from build123d import *

# Parameters (mm, degrees)
SKETCH1_W           = 127
SKETCH1_H           = 127
BOSS_EXTRUDE1_DEPTH = 127
SKETCH13_W          = 43.18
SKETCH13_H          = 43.18
SKETCH13_W_2        = 29.718
SKETCH13_H_2        = 29.718
BOSS_EXTRUDE7_DEPTH = 6.35
SKETCH29_R          = 40.64
CUT_EXTRUDE10_DEPTH = 6.35
SKETCH27_W          = 43.18
SKETCH27_H          = 43.18
SKETCH27_W_2        = 29.718
SKETCH27_H_2        = 29.718
BOSS_EXTRUDE8_DEPTH = 6.35
SKETCH28_R          = 40.64
CUT_EXTRUDE11_DEPTH = 6.35


with BuildPart() as part:
    # Sketch1 → Boss-Extrude1 (new body)
    with BuildSketch(Plane.XY):
        Rectangle(SKETCH1_W, SKETCH1_H)
    extrude(amount=BOSS_EXTRUDE1_DEPTH)

    # Sketch13 → Boss-Extrude7 (add)
    with BuildSketch(Plane(origin=(0, 0, 0), x_dir=(-1, 0, 0), z_dir=(0, 0, -1))):
        with Locations((-41.91, 41.91)):
            Rectangle(SKETCH13_W, SKETCH13_H)
        with Locations((-41.91, -41.91)):
            Rectangle(SKETCH13_W, SKETCH13_H)
        with Locations((41.91, 41.91)):
            Rectangle(SKETCH13_W, SKETCH13_H)
        with Locations((41.91, -41.91)):
            Rectangle(SKETCH13_W, SKETCH13_H)
        with Locations((-48.641, 0)):
            Rectangle(SKETCH13_W_2, SKETCH13_H_2)
        with Locations((0, -48.641)):
            Rectangle(SKETCH13_W_2, SKETCH13_H_2)
        with Locations((48.641, 0)):
            Rectangle(SKETCH13_W_2, SKETCH13_H_2)
        with Locations((0, 48.641)):
            Rectangle(SKETCH13_W_2, SKETCH13_H_2)
    extrude(amount=BOSS_EXTRUDE7_DEPTH)

    # Sketch29 → Cut-Extrude10 (cut)
    with BuildSketch(Plane(origin=(0, 0, 0), x_dir=(-1, 0, 0), z_dir=(0, 0, -1))):
        Circle(SKETCH29_R)
    extrude(amount=CUT_EXTRUDE10_DEPTH, mode=Mode.SUBTRACT)

    # Sketch27 → Boss-Extrude8 (add)
    with BuildSketch(Plane(origin=(63.5, 0, 0), x_dir=(0, 0, -1), z_dir=(1, 0, 0))):
        with Locations((-105.41, 41.91)):
            Rectangle(SKETCH27_W, SKETCH27_H)
        with Locations((-105.41, -41.91)):
            Rectangle(SKETCH27_W, SKETCH27_H)
        with Locations((-21.59, 41.91)):
            Rectangle(SKETCH27_W, SKETCH27_H)
        with Locations((-21.59, -41.91)):
            Rectangle(SKETCH27_W, SKETCH27_H)
        with Locations((-112.141, -0.254760407)):
            Rectangle(SKETCH27_W_2, SKETCH27_H_2)
        with Locations((-63.013602448, -48.641)):
            Rectangle(SKETCH27_W_2, SKETCH27_H_2)
        with Locations((-14.859, -0.254760407)):
            Rectangle(SKETCH27_W_2, SKETCH27_H_2)
        with Locations((-63.013602448, 48.641)):
            Rectangle(SKETCH27_W_2, SKETCH27_H_2)
    extrude(amount=BOSS_EXTRUDE8_DEPTH)

    # Sketch28 → Cut-Extrude11 (cut)
    with BuildSketch(Plane(origin=(63.5, 0, 0), x_dir=(0, 0, -1), z_dir=(1, 0, 0))):
        with Locations((-63.5, 0)):
            Circle(SKETCH28_R)
    extrude(amount=CUT_EXTRUDE11_DEPTH, mode=Mode.SUBTRACT)


solid = part.part
Can you work these out from the model? Positions are in its coordinate system, mm. A direction names the side the tool comes from. Give positions to 0.01 mm unless a question says otherwise; leave off trailing zeros. Order: outer loops, then holes, each group sorted by start corner. A loop starts at its lowest first (then second) coordinate and runs counter-clockwise, first axis right, second up. Notation, with made-up numbers: M -3,86 L 48,86 A21 cw 48,107 Z; hole C 36,22 d3. An arc over 180 degrees is marked long. One line per item, written item: value.
Item 1: If we section it at C-C on z = 54: Write out the boundary of the cut face in (x, y).
Verdict:
outline: M -63.5,-63.5 L 69.85,-63.5 L 69.85,-39.51 L 63.5,-39.51 L 63.5,39.51 L 69.85,39.51 L 69.85,63.5 L -63.5,63.5 Z
Item 2: For pin 1 (3 mm diameter, centred on y = -38, z = -4, fed in from +X); pin 2 (12 mm diameter, centred on x = 15.5, y = 22.5, fed in from -Z), each with a flat end and sliding along its axis, tell me the tip position at first contact or that it passes through.
Verdict:
pin 1: x = 63.5
pin 2: z = 0
Item 3: If we mould it in two halves opening along Y, with no side actions, what happens to faces 5 (the face through (-49, 20.32, -3)), 6 (the face through (69.85, -50, 63))? For each: pulls with the +Y half, pulls with the -Y half, needs draft (parallel to the pull), parting line crosses it, or undercut.
Verdict:
face 5: undercut
face 6: needs draft
Item 4: If we section it at A-A on y = -9.5: Write out the boundary of the cut face in (x, z).
Verdict:
outline: M -63.5,-6.35 L -39.51,-6.35 L -39.51,0 L 39.51,0 L 39.51,-6.35 L 63.5,-6.35 L 63.5,0 L 69.85,0 L 69.85,23.99 L 63.5,23.99 L 63.5,103.01 L 69.85,103.01 L 69.85,127 L -63.5,127 Z
Item 5: If we section it at D-D on y = 26: Write out the boundary of the cut face in (x, z).
Verdict:
outline: M -63.5,-6.35 L -31.23,-6.35 L -31.23,0 L 31.23,0 L 31.23,-6.35 L 63.5,-6.35 L 63.5,0 L 69.85,0 L 69.85,32.27 L 63.5,32.27 L 63.5,94.73 L 69.85,94.73 L 69.85,127 L -63.5,127 Z
Item 6: Please list where these lines run through material, in increasing order: line 1 (Z direction, x = 4, y = 24); line 2 (X direction, y = 3.5, z = 59).
Verdict:
line 1: 0 to 127
line 2: -63.5 to 63.5
Item 7: If we section it at B-B on x = 23.5: Write out the boundary of the cut face in (y, z), and give its area (3 significant figures).
Verdict:
outline: M -63.5,-6.35 L -33.16,-6.35 L -33.16,0 L 33.16,0 L 33.16,-6.35 L 63.5,-6.35 L 63.5,127 L -63.5,127 Z
area: 16,500 mm2
Item 8: For faces 1 (the face through (-0.21, 40.64, -3.13)), 2 (the face through (51, 14.859, -3)), 3 (the face through (67, 20.32, 113)), 4 (the face through (-20.32, -50, -3)), which set-ups out of +Z, -Z, +X, -X, +Y, -Y let a thin tool reach every point of the face, with its end or its side?
Verdict:
face 1: -Z
face 2: -Z, +X, -X
face 3: +Z, -Z, +X
face 4: -Z, +Y, -Y
